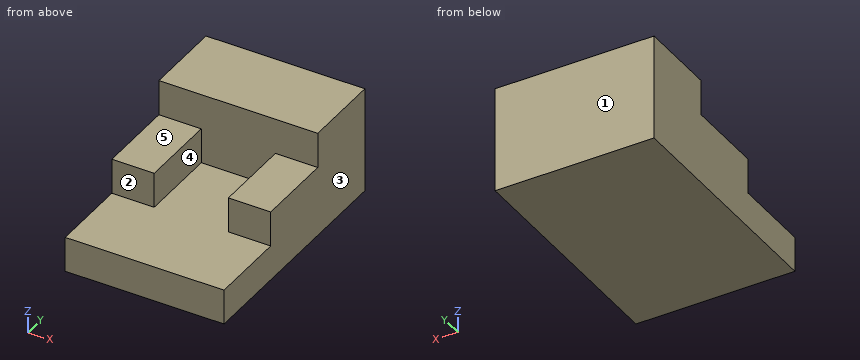
from build123d import *

# Parameters (mm, degrees)
F0_W     = 38.1
F0_H     = 19.05
F1_DEPTH = 25.4
F2_W     = 38.1
F2_H     = 38.1
F3_DEPTH = 8.4328
F4_W     = 10.16
F4_H     = 19.05
F5_DEPTH = 8.4582
F6_DEPTH = 8.46328


with BuildPart() as f1:
    # F0 (on Top) → F1 (new body)
    with BuildSketch(Plane.XY):
        Rectangle(F0_W, F0_H)
    extrude(amount=F1_DEPTH)

    # F2 (on Top) → F3 (join)
    with BuildSketch(Plane.XY):
        with Locations((0, -28.427749)):
            Rectangle(F2_W, F2_H)
    extrude(amount=F3_DEPTH)

    # F4 (on face) → F5 (join)
    with BuildSketch(Plane.XY.offset(8.4328)):
        with Locations((-13.97, -19.05)):
            Rectangle(F4_W, F4_H)
    extrude(amount=F5_DEPTH)

    # F4 (on face) → F6 (join)
    with BuildSketch(Plane.XY.offset(8.4328)):
        with Locations((13.97, -19.05)):
            Rectangle(F4_W, F4_H)
    extrude(amount=F6_DEPTH)


solid = f1.part
Design review of the part built by this model. Coordinates are the model's own, in mm. Face numbers are marked on the shaded views. A direction names the side the tool comes from. Round coordinates to 2 decimals unless told otherwise and drop trailing zeros. Write each loop counter-clockwise with the first axis right and the second up, starting at its lowest first coordinate (ties: lowest second). Pieces come first, ordered by that corner, then holes. Notation, with made-up numbers: M 0,24.5 L 36,24.5 A20 ccw 36,49.5 Z; hole C 14.5,-40 d11. An arc over 180 degrees is marked long. One line per item, written item: value. Start each with the question number.
1. Draft analysis for pull direction X (two halves, no side actions). For the marked faces 3, 4 and 5, state which applies: pulls with the +X half, pulls with the -X half, needs draft (parallel to the pull), parting line crosses it, or undercut.
2. Take a section at A-A on y = -12. State the section outline as (x, z) points, then the cut area to 3 significant figures.
3. Take a section at C-C on z = 22. State the section outline as (x, y) points (3 decimals).
4. To check wall thickness, follow probe 1 along X at (y, z) = (-14.5, 11.75); probe 2 along Z at (x, y) = (14, -20); probe 3 along Z at (x, y) = (-6, -37.5). State the ranges of each line that lie inside material, in increasing order. Write a range as from..to.
5. Take a section at D-D on x = -0.5. State the section outline as (y, z) points (3 decimals).
6. For the marked faces 1 and 2, list the 3-axis set-ups (+Z, -Z, +X, -X, +Y, -Y) from which the entire face can be reached by the end or side of a thin tool; tool diameter is ignored.
7. Clearance check with flat-ended pins moving along their axes: P1, Ø2, axis at y = -16.5, z = 17.5, coming from the -X side; P2, Ø11.5, axis at x = 4.5, y = -29, coming from the +Z side; P3, Ø8.5, axis at x = 0, z = 15, coming from the -Y side (3 decimals); P4, Ø2.5, axis at x = -15.5, z = 12, coming from the -Y side (3 decimals). State where each tip first meets the part, or that it passes through.
8. Take a section at B-B on x = -15.5. State the section outline as (y, z) points (3 decimals), then the cut area to 3 significant figures.
Computed:
1. face 3: pulls with the +X half
1. face 4: undercut
1. face 5: needs draft
2. outline: M -19.05,0 L 19.05,0 L 19.05,16.9 L 8.89,16.9 L 8.89,8.43 L -8.89,8.43 L -8.89,16.89 L -19.05,16.89 Z
2. area: 493 mm²
3. outline: M -19.05,-9.525 L 19.05,-9.525 L 19.05,9.525 L -19.05,9.525 Z
4. probe 1: x = -19.05..-8.89, 8.89..19.05
4. probe 2: z = 0..16.9
4. probe 3: z = 0..8.43
5. outline: M -47.478,0 L 9.525,0 L 9.525,25.4 L -9.525,25.4 L -9.525,8.433 L -47.478,8.433 Z
6. face 1: +Z, -Z, +X, -X, +Y
6. face 2: +Z, +X, -X, -Y
7. P1: stops at x = -19.05
7. P2: stops at z = 16.9
7. P3: stops at y = -9.525
7. P4: stops at y = -28.575
8. outline: M -47.478,0 L 9.525,0 L 9.525,25.4 L -9.525,25.4 L -9.525,16.891 L -28.575,16.891 L -28.575,8.433 L -47.478,8.433 Z
8. area: 965 mm²
